Here's the drawing with two shaded views (mm, measured from the low corner). I have some questions. Coordinates: 2 decimals unless noted, no trailing zeros. Write each loop counter-clockwise with the first axis right and the second up, starting at its lowest first coordinate (ties: lowest second). Pieces come first, ordered by that corner, then holes.
Item 1: I want a section at B-B on x = 1.5. State how many separate pieces and enclosed holes the cut face has.
Item 2: I want a section at A-A on y = 12.7. Please give me the cut outline in (x, z), then the cut area to 3 significant figures.
Item 3: Thinking about a two-plate mould opening in Y: for the marked faces 1, 2 and 3, which applies, +Y half, -Y half, draft (parallel to the pull), parting line (faces both ways), or undercut?
Item 4: If I drill on probe 1 along Y at (x, z) = (3.25, 5.5) (1 decimal); probe 2 along X at (y, z) = (12.75, 6); probe 3 along Y at (x, z) = (3.75, 6.25) (1 decimal), over which ranges is the centre line in solid material (lowest first)?
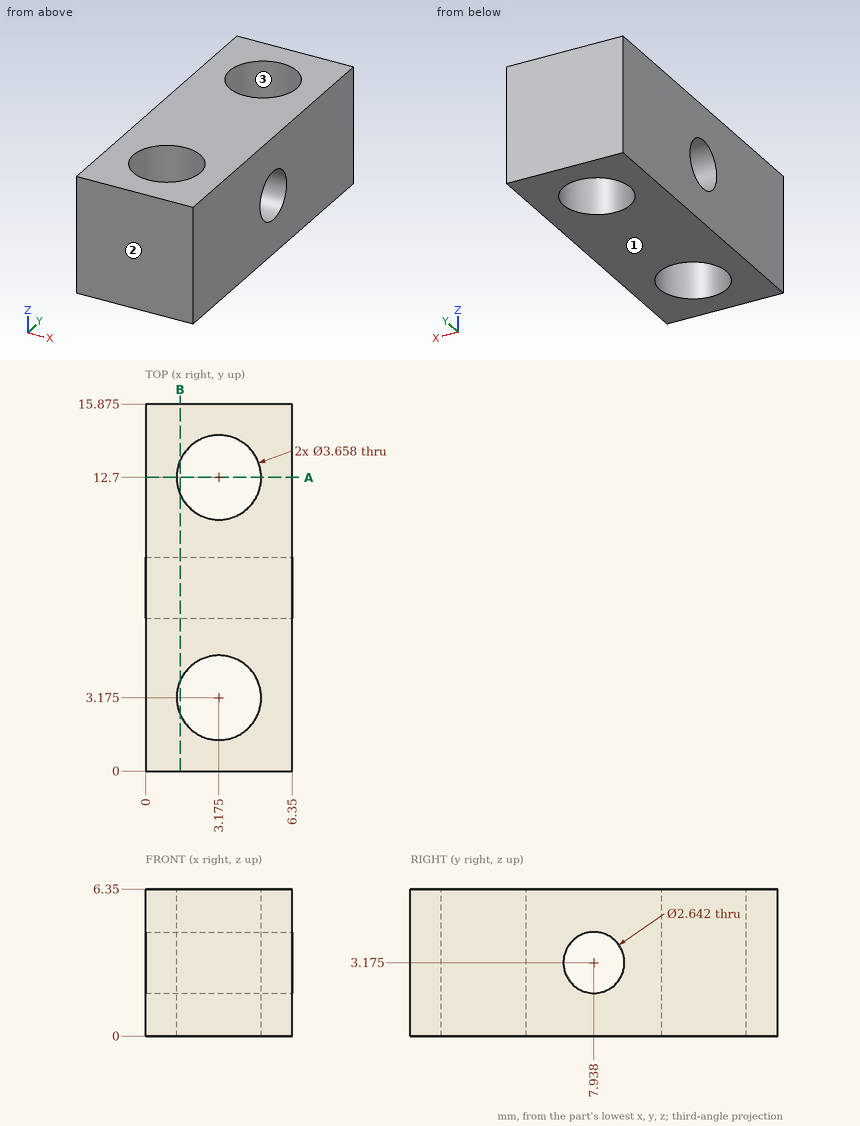
Response values:
1. separate pieces: 3
1. enclosed holes: 1
2. outline: (0, 0) - (1.35, 0) - (1.35, 6.35) - (0, 6.35) - close; (5, 0) - (6.35, 0) - (6.35, 6.35) - (5, 6.35) - close
2. area: 17.1 mm2
3. face 1: draft
3. face 2: -Y half
3. face 3: undercut
4. probe 1: y = 0 to 1.3, 5 to 10.9, 14.5 to 15.9
4. probe 2: x = 0 to 1.35, 5 to 6.35
4. probe 3: y = 0 to 1.4, 4.9 to 11, 14.4 to 15.9
